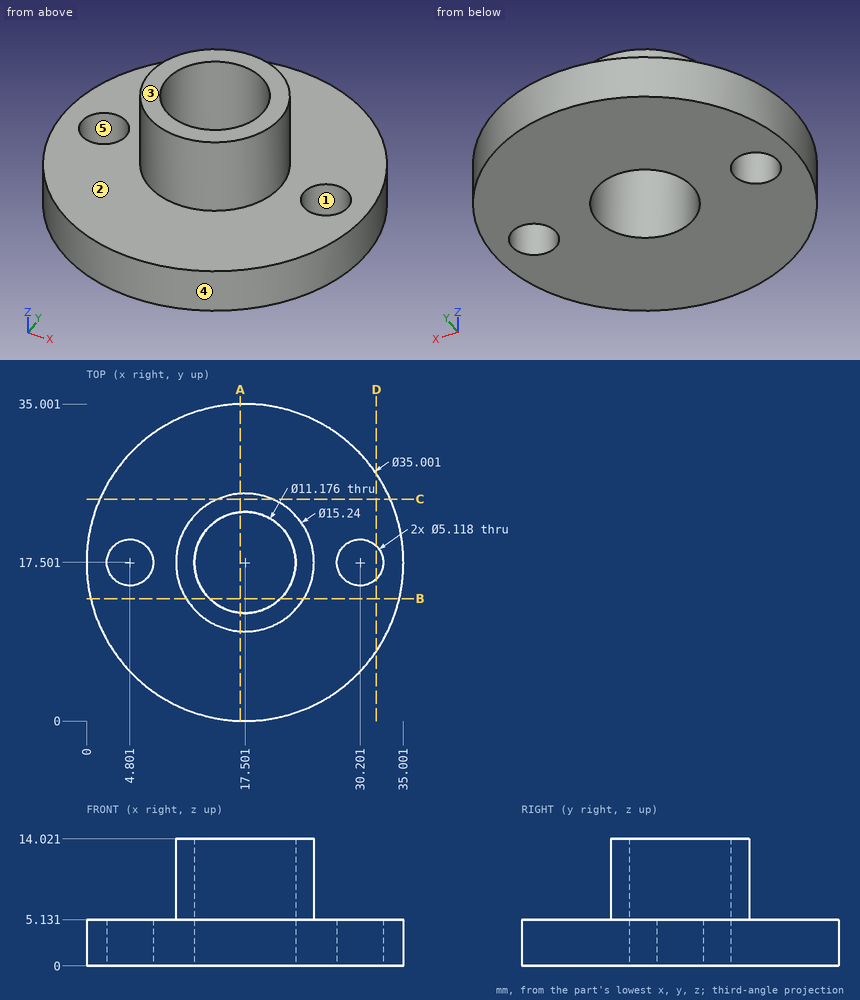
Part print with two shaded views. Sizes in mm from the minimum x, y, z corner. A direction names the side the tool comes from. Coordinates: 2 decimals unless noted, no trailing zeros. Order: outer loops, then holes, each group sorted by start corner. A loop starts at its lowest first (then second) coordinate and runs counter-clockwise, first axis right, second up. Notation, with made-up numbers: (89.25, 12) - (144.25, 12) arc R20 cw to (144.25, 22) - close; hole circle Ø7 at (-8, 7). An arc over 180 degrees is marked (long way). Write item = value, one per line. Start each with the question number.
1) Saw through at A-A on x = 17. Write the cut outline in (y, z) (1 decimal), then the cut area to 3 significant figures.
2) Flat gauge pins, fed straight in: pin 1 Ø10 at (x, y) = (17.5, 17.5) entering from -Z; pin 2 Ø3 at (x, y) = (4, 7) entering from +Z; pin 3 Ø5 at (y, z) = (19.5, 9.5) entering from -X; pin 4 Ø6 at (x, z) = (26.5, 10.5) entering from -Y. Where does each tip first touch, or does it go through?
3) Saw through at B-B on y = 13.5. Write the cut outline in (x, z) (1 decimal).
4) 3-axis set-ups, long thin cutter, end or side, ignore diameter. For the marked faces 1 and 2: which of +Z, -Z, +X, -X, +Y, -Y reach the whole face in a straight line?
5) Two-plate mould, pull along Y, no slides. Class the marked faces 3, 4 and 5: pulls with the +Y half, pulls with the -Y half, needs draft (parallel to the pull), parting line crosses it, or undercut.
6) Wall check: line 1 along Z through (x, y) = (17.5, 3); line 2 along Y through (x, z) = (16, 12.5). Give the ranges that are in metal, low to high. Write a range as from..to.
7) Saw through at D-D on x = 32. Write the cut outline in (y, z).
8) Saw through at C-C on y = 24.5. Write the cut outline in (x, z).
From the geometry:
q1.outline = (0, 0) - (11.9, 0) - (11.9, 14) - (9.9, 14) - (9.9, 5.1) - (0, 5.1) - close; (23.1, 0) - (35, 0) - (35, 5.1) - (25.1, 5.1) - (25.1, 14) - (23.1, 14) - close
q1.area = 159 mm^2
q2.pin_1 = through
q2.pin_2 = 5.13
q2.pin_3 = 9.88
q2.pin_4 = 12.8
q3.outline = (0.5, 0) - (13.6, 0) - (13.6, 14) - (11, 14) - (11, 5.1) - (0.5, 5.1) - close; (21.4, 0) - (34.5, 0) - (34.5, 5.1) - (24, 5.1) - (24, 14) - (21.4, 14) - close
q4.face_1 = +Z, -Z
q4.face_2 = +Z
q5.face_3 = needs draft
q5.face_4 = parting line crosses it
q5.face_5 = undercut
q6.line_1 = 0..5.13
q6.line_2 = 10.03..12.12, 22.88..24.97
q7.outline = (7.7, 0) - (15.68, 0) - (15.68, 5.13) - (7.7, 5.13) - close; (19.32, 0) - (27.3, 0) - (27.3, 5.13) - (19.32, 5.13) - close
q8.outline = (1.46, 0) - (33.54, 0) - (33.54, 5.13) - (20.51, 5.13) - (20.51, 14.02) - (14.49, 14.02) - (14.49, 5.13) - (1.46, 5.13) - close
